from build123d import *

# Parameters (mm, degrees)
SKETCH1_R           = 6
SKETCH1_R_2         = 1.5
BOSS_EXTRUDE1_DEPTH = 1
SKETCH3_R           = 9.5
SKETCH3_R_2         = 8
BOSS_EXTRUDE2_DEPTH = 1


with BuildPart() as part:
    # Sketch1 → Boss-Extrude1 (new body)
    with BuildSketch(Plane(origin=(0, 0, 0), x_dir=(1, 0, 0), z_dir=(0, 1, 0))):
        with BuildLine():
            ThreePointArc((10.722201854, 4.157449627), (10.598848399, 5.689199117), (11.333854237, 7.038731997))
            ThreePointArc((11.333854237, 7.038731997), (11.345969357, 11.281355386), (7.103345968, 11.293470506))
            ThreePointArc((7.103345968, 11.293470506), (5.749637406, 10.566183969), (4.218617379, 10.698283386))
            ThreePointArc((4.218617379, 10.698283386), (0.032838952, 11.499953113), (-4.157449627, 10.722201854))
            ThreePointArc((-4.157449627, 10.722201854), (-5.689199117, 10.598848399), (-7.038731997, 11.333854237))
            ThreePointArc((-7.038731997, 11.333854237), (-11.281355386, 11.345969357), (-11.293470506, 7.103345968))
            ThreePointArc((-11.293470506, 7.103345968), (-10.566183969, 5.749637406), (-10.698283386, 4.218617379))
            ThreePointArc((-10.698283386, 4.218617379), (-11.499953113, 0.032838952), (-10.722201854, -4.157449627))
            ThreePointArc((-10.722201854, -4.157449627), (-10.598848399, -5.689199117), (-11.333854237, -7.038731997))
            ThreePointArc((-11.333854237, -7.038731997), (-11.345969357, -11.281355386), (-7.103345968, -11.293470506))
            ThreePointArc((-7.103345968, -11.293470506), (-5.749637406, -10.566183969), (-4.218617379, -10.698283386))
            ThreePointArc((-4.218617379, -10.698283386), (-0.032838952, -11.499953113), (4.157449627, -10.722201854))
            ThreePointArc((4.157449627, -10.722201854), (5.689199117, -10.598848399), (7.038731997, -11.333854237))
            ThreePointArc((7.038731997, -11.333854237), (11.281355386, -11.345969357), (11.293470506, -7.103345968))
            ThreePointArc((11.293470506, -7.103345968), (10.566183969, -5.749637406), (10.698283386, -4.218617379))
            ThreePointArc((10.698283386, -4.218617379), (11.499953113, -0.032838952), (10.722201854, 4.157449627))
        make_face()
        Circle(SKETCH1_R, mode=Mode.SUBTRACT)
        with Locations((9.218600102, 9.166101251)):
            Circle(SKETCH1_R_2, mode=Mode.SUBTRACT)
        with Locations((9.166101251, -9.218600102)):
            Circle(SKETCH1_R_2, mode=Mode.SUBTRACT)
        with Locations((-9.166101251, 9.218600102)):
            Circle(SKETCH1_R_2, mode=Mode.SUBTRACT)
        with Locations((-9.218600102, -9.166101251)):
            Circle(SKETCH1_R_2, mode=Mode.SUBTRACT)
    extrude(amount=BOSS_EXTRUDE1_DEPTH)

    # Sketch3 → Boss-Extrude2 (add)
    with BuildSketch(Plane(origin=(0, 0, 0), x_dir=(1, 0, 0), z_dir=(0, 1, 0))):
        Circle(SKETCH3_R)
        Circle(SKETCH3_R_2, mode=Mode.SUBTRACT)
    extrude(amount=-BOSS_EXTRUDE2_DEPTH)


solid = part.part
Could you check a few things on this model? Use its own coordinates, in mm. A direction names the side the tool comes from. Give positions to 0.01 mm unless a question says otherwise; leave off trailing zeros. Order: outer loops, then holes, each group sorted by start corner. A loop starts at its lowest first (then second) coordinate and runs counter-clockwise, first axis right, second up.
1. For pin 1 (5 mm diameter, centred on x = 3.5, z = -3.5, fed in from -Y); pin 2 (1 mm diameter, centred on x = -8.5, y = -1, fed in from +Z), each with a flat end and sliding along its axis, tell me the tip position at first contact or that it passes through.
Answers below:
pin 1: stops at y = 0
pin 2: stops at z = 5.12
2. Which directions (+Z, -Z, +X, -X, +Y, -Y) give clear straight access to the entire face, cutting with the end or side of a thin tool? Please do faces 4 (the flat face through (-2, 0, -6)), 5 (the cylindrical face through (9.97, 0.49, 7.95)).
Answers below:
face 4: -Y
face 5: +Y, -Y
3. I need wall thicknesses on L1, parallel to X at y = 0.8, z = 0; L2, parallel to X at y = 0.2, z = 9.75. Which ranges of each line are inside material? Lowest first, please.
Answers below:
L1: x = -11.5 to -6, 6 to 11.5
L2: x = -12.16 to -10.6, -7.84 to 7.76, 10.57 to 12.12
4. Suppose I cut it at C-C (y = 0.5). Write out the boundary of the cut face in (x, z), plus the area to 3 significant figures.
Answers below:
outline: (-11.33, 7.04) arc R2.69 cw to (-10.72, 4.16) arc R11.5 ccw to (-10.7, -4.22) arc R2.69 cw to (-11.29, -7.1) arc R3 ccw to (-7.04, -11.33) arc R2.69 cw to (-4.16, -10.72) arc R11.5 ccw to (4.22, -10.7) arc R2.69 cw to (7.1, -11.29) arc R3 ccw to (11.33, -7.04) arc R2.69 cw to (10.72, -4.16) arc R11.5 ccw to (10.7, 4.22) arc R2.69 cw to (11.29, 7.1) arc R3 ccw to (7.04, 11.33) arc R2.69 cw to (4.16, 10.72) arc R11.5 ccw to (-4.22, 10.7) arc R2.69 cw to (-7.1, 11.29) arc R3 ccw to start; hole circle Ø3 at (-9.22, 9.17); hole circle Ø3 at (-9.17, -9.22); hole circle Ø12 at (0, 0); hole circle Ø3 at (9.17, 9.22); hole circle Ø3 at (9.22, -9.17)
area: 375 mm2
5. Suppose I cut it at A-A (x = 0). Write out the boundary of the cut face in (y, z).
Answers below:
outline: (-1, -9.5) - (0, -9.5) - (0, -11.5) - (1, -11.5) - (1, -6) - (0, -6) - (0, -8) - (-1, -8) - close; (-1, 8) - (0, 8) - (0, 6) - (1, 6) - (1, 11.5) - (0, 11.5) - (0, 9.5) - (-1, 9.5) - close
6. Thinking about a two-plate mould opening in Z: for faces 1 (the cylindrical face through (-5.7, 0.5, -10.6)), 2 (the cylindrical face through (5.7, 0.5, 10.6)), 3 (the cylindrical face through (-8.412, 0.493, 7.901)), which applies, +Z half, -Z half, draft (parallel to the pull), parting line (faces both ways), or undercut?
Answers below:
face 1: -Z half
face 2: +Z half
face 3: undercut
7. Suppose I cut it at B-B (z = 0). Write out the boundary of the cut face in (x, y).
Answers below:
outline: (-11.5, 0) - (-9.5, 0) - (-9.5, -1) - (-8, -1) - (-8, 0) - (-6, 0) - (-6, 1) - (-11.5, 1) - close; (6, 0) - (8, 0) - (8, -1) - (9.5, -1) - (9.5, 0) - (11.5, 0) - (11.5, 1) - (6, 1) - close
